The model under review builds one solid part; all positions refer to its coordinate system, in mm. Round coordinates to 2 decimals unless told otherwise and drop trailing zeros. Order: outer loops, then holes, each group sorted by start corner. A loop starts at its lowest first (then second) coordinate and runs counter-clockwise, first axis right, second up. Notation, with made-up numbers: (87, 30.5) -> (124, 30.5) arc R12 ccw to (124, 49.5) -> close; hole circle Ø9 at (53, 37.5). An arc over 180 degrees is marked (long way). Return JSON: item names as keys, results as strings. Group by question number.
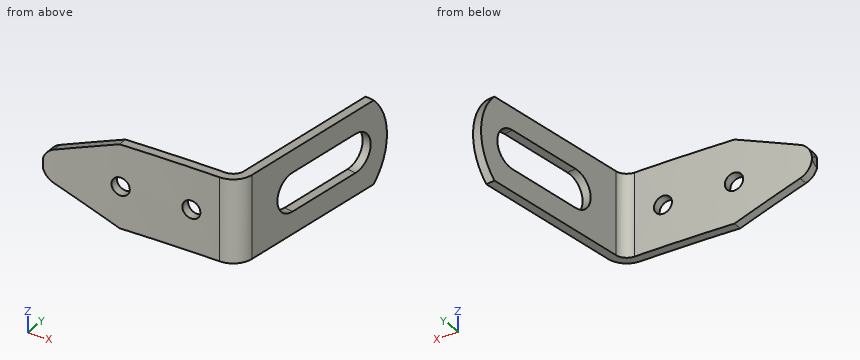
from build123d import *

# Parameters (mm, degrees)
EXTRUSION1_DEPTH             = 7
ENL_V_MAT_EXTRU_1_DEPTH      = 37.038682389
ENL_V_MAT_EXTRU_2_DEPTH      = 32.917281873
ENL_V_MAT_EXTRU_2_DEPTH_BACK = 2.378196501


with BuildPart() as part:
    # Esquisse1 → Extrusion1 (new body, symmetric)
    with BuildSketch(Plane.XY):
        with BuildLine():
            Line((0.403563953, 3.024571148), (4.232204488, 31.718897288))
            Line((4.232204488, 31.718897288), (2.745381178, 31.917281873))
            Line((2.745381178, 31.917281873), (-1.083259357, 3.222955733))
            ThreePointArc((-1.083259357, 3.222955733), (-1.742171349, 1.988036214), (-3.049340089, 1.487535348))
            ThreePointArc((-3.049340089, 1.487535348), (-17.587736804, 1.085119824), (-32.099393733, 0.116238776))
            Line((-32.099393733, 0.116238776), (-31.9703077, -1.378196501))
            ThreePointArc((-31.9703077, -1.378196501), (-17.51700864, -0.413211757), (-3.037077327, -0.012414526))
            ThreePointArc((-3.037077327, -0.012414526), (-0.749532032, 0.863461989), (0.403563953, 3.024571148))
        make_face()
    extrude(amount=EXTRUSION1_DEPTH, both=True)

    # Esquisse2 → Enlèv. mat.-Extru.1 (cut, through all)
    with BuildSketch(Plane(origin=(0, 0, 0), x_dir=(0, 0, -1), z_dir=(0.99121554, -0.13225639, 0))):
        with BuildLine():
            Line((-3.25, 11.75), (-3.25, 25.25))
            ThreePointArc((-3.25, 25.25), (0, 28.5), (3.25, 25.25))
            Line((3.25, 25.25), (3.25, 11.75))
            ThreePointArc((3.25, 11.75), (0, 8.5), (-3.25, 11.75))
        make_face()
        with BuildLine():
            Line((-7, 32), (-7, 29.141428429))
            ThreePointArc((-7, 29.141428429), (0, 32), (7, 29.141428429))
            Line((7, 29.141428429), (7, 32))
            ThreePointArc((7, 32), (0, 34.206555616), (-7, 32))
        make_face()
    extrude(amount=-ENL_V_MAT_EXTRU_1_DEPTH, mode=Mode.SUBTRACT)

    # Esquisse3 → Enlèv. mat.-Extru.2 (cut, two sides)
    with BuildSketch(Plane(origin=(0, 0, 0), x_dir=(1, 0, 0), z_dir=(0, 1, 0))) as enl_v_mat_extru_2_sk:
        with BuildLine():
            Line((-19.599393733, 7), (-30.206517298, 2.788239124))
            ThreePointArc((-30.206517298, 2.788239124), (-32.099393733, 0), (-30.206517298, -2.788239124))
            Line((-30.206517298, -2.788239124), (-19.599393733, -7))
            Line((-19.599393733, -7), (-32.099393733, -7))
            ThreePointArc((-32.099393733, -7), (-36.715166839, 0), (-32.099393733, 7))
            Line((-32.099393733, 7), (-19.599393733, 7))
        make_face()
    extrude(amount=ENL_V_MAT_EXTRU_2_DEPTH, mode=Mode.SUBTRACT)
    extrude(enl_v_mat_extru_2_sk.sketch, amount=-ENL_V_MAT_EXTRU_2_DEPTH_BACK, mode=Mode.SUBTRACT)

    # Esquisse4 → Enlèvement de matière-Révolution1 (revolve, cut)
    with BuildSketch(Plane.XY, mode=Mode.PRIVATE) as enl_vement_de_mati_re_r_volution1_sk:
        Polygon((-20.993708492, 29.083821309), (-19.397261786, -1.378196501), (-20.899320305, -1.378196501), (-22.495767011, 29.083821309), align=None)
    revolve(enl_vement_de_mati_re_r_volution1_sk.sketch.rotate(Axis((0, -371.5, 0), (-0.052335956, 0.998629535, 0)), 180), axis=Axis((0, -371.5, 0), (-0.052335956, 0.998629535, 0)), mode=Mode.SUBTRACT)  # turned: the seam where the file's is

    # Esquisse5 → Enlèvement de matière-Révolution2 (revolve, cut)
    with BuildSketch(Plane.XY, mode=Mode.PRIVATE) as enl_vement_de_mati_re_r_volution2_sk:
        Polygon((-9.530265596, 11.845167183), (-9.263238962, -0.902551216), (-7.763567936, -0.871137586), (-8.029936549, 11.845167183), align=None)
    revolve(enl_vement_de_mati_re_r_volution2_sk.sketch.rotate(Axis((0, -371.5, 0), (-0.02094242, 0.999780683, 0)), 180), axis=Axis((0, -371.5, 0), (-0.02094242, 0.999780683, 0)), mode=Mode.SUBTRACT)  # turned: the seam where the file's is


solid = part.part
Item 1: Consider section C-C on x = -14.5. State the section outline as (y, z) points.
Item 2: Consider section A-A on y = 18. State the section outline as (x, z) points, plus the area to 3 significant figures.
Item 3: Wall thickness on line 1 along Y through (x, z) = (-3.5, -5.25); line 2 along X through (y, z) = (17, -4) (3 decimals); line 3 along X through (y, z) = (3.5, -4): over which ranges is each line inside the solid? List them lowest first.
Item 4: Consider section B-B on z = 3.75. State the section outline as (x, y) points, plus the area to 3 significant figures.
Item 5: Insertion check: pin 1 Ø6 at (y, z) = (6.5, -0.5) entering from +X; pin 2 Ø1.5 at (y, z) = (4.5, -2) entering from -X; pin 3 Ø8 at (y, z) = (26.5, -1) entering from +X. Each pin has a flat end and moves straight along its axis. Give the tip position at first contact, or say it passes through.
Item 6: Consider section D-D on z = -5.75. State the section outline as (x, y) points.
Values:
{
 "1": {"outline": "(-0.28, -7) -> (1.22, -7) -> (1.22, 7) -> (-0.28, 7) -> close"},
 "2": {"outline": "(0.89, -7) -> (2.4, -7) -> (2.4, -3.25) -> (0.89, -3.25) -> close; (0.89, 3.25) -> (2.4, 3.25) -> (2.4, 7) -> (0.89, 7) -> close", "area": "11.3 mm^2"},
 "3": {"line 1": "-0.02 to 1.48", "line 2": "0.755 to 2.268", "line 3": "-1.05 to 0.47"},
 "4": {"outline": "(-27.78, -1.04) arc R371.5 cw to (-3.04, -0.01) arc R3.5 ccw to (0.4, 3.02) -> (4.14, 31) -> (2.65, 31.19) -> (-1.08, 3.22) arc R2 cw to (-3.05, 1.49) arc R373 ccw to (-27.78, 0.46) -> close", "area": "85.4 mm^2"},
 "5": {"pin 1": "x = 1.21", "pin 2": "x = -1.01", "pin 3": "x = 4.07"},
 "6": {"outline": "(-22.75, -0.7) arc R371.5 cw to (-3.04, -0.01) arc R3.5 ccw to (0.4, 3.02) -> (3.99, 29.92) -> (2.5, 30.11) -> (-1.08, 3.22) arc R2 cw to (-3.05, 1.49) arc R373 ccw to (-22.75, 0.81) -> close"}
}
